Here's the drawing with two shaded views (mm, measured from the low corner). I have some questions. A direction names the side the tool comes from. Round coordinates to 2 decimals unless told otherwise and drop trailing zeros. Order: outer loops, then holes, each group sorted by start corner. A loop starts at its lowest first (then second) coordinate and runs counter-clockwise, first axis right, second up. Notation, with made-up numbers: (49.25, 60.5) -> (78.25, 60.5) arc R14 cw to (78.25, 84.5) -> close; hole circle Ø8 at (-32.75, 36). An arc over 180 degrees is marked (long way). One line per question, with ' | ' between items.
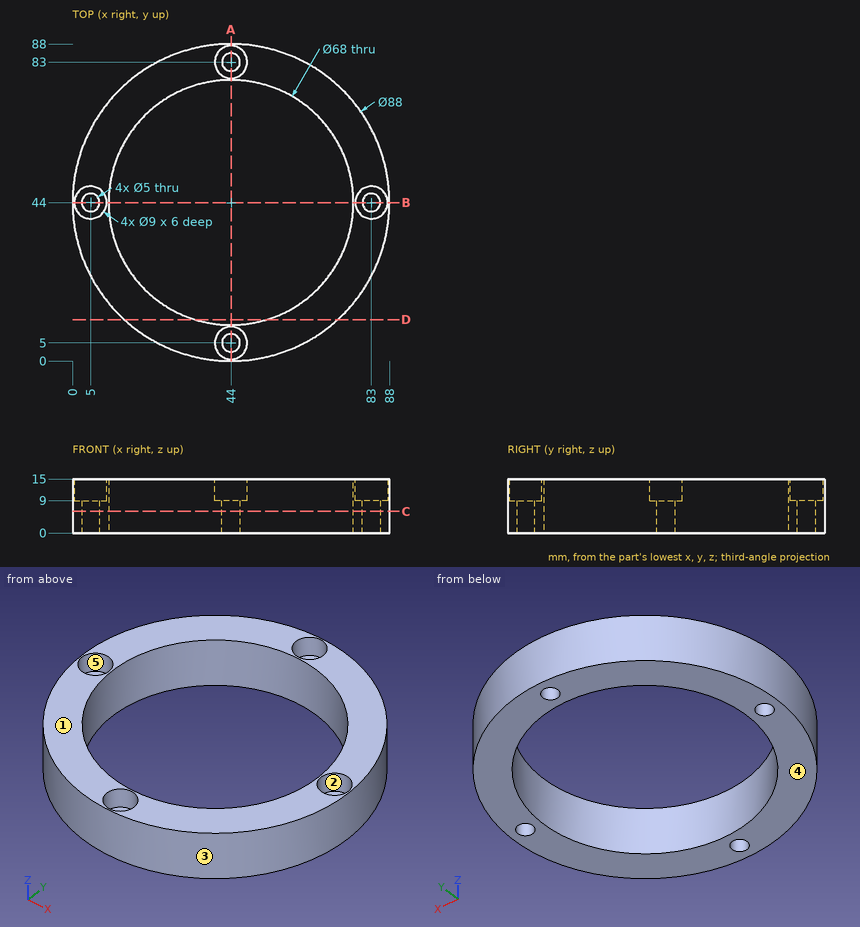
1. If we mould it in two halves opening along X, with no side actions, what happens to the marked faces 3, 4 and 5? For each: pulls with the +X half, pulls with the -X half, needs draft (parallel to the pull), parting line crosses it, or undercut.
From the geometry:
face 3: parting line crosses it | face 4: needs draft | face 5: undercut
2. I'm going to push flat-ended pins straight in: pin 1 (4.5 mm diameter, centred on x = 44.5, y = 85, fed in from +Z); pin 2 (4.5 mm diameter, centred on x = 83, y = 44, fed in from +Z); pin 3 (1 mm diameter, centred on y = 64.5, z = 8, fed in from +X); pin 4 (5 mm diameter, centred on x = 34, z = 6.5, fed in from +Y). Where does each tip first touch, or does it pass through?
From the geometry:
pin 1: stops at z = 9 | pin 2: passes through | pin 3: stops at x = 83.19 | pin 4: stops at y = 87.36
3. I want a section at A-A on x = 44. List the corners of the cut face in (y, z) for me.
From the geometry:
outline: (0, 0) -> (2.5, 0) -> (2.5, 9) -> (0.5, 9) -> (0.5, 15) -> (0, 15) -> close; (7.5, 0) -> (10, 0) -> (10, 15) -> (9.5, 15) -> (9.5, 9) -> (7.5, 9) -> close; (78, 0) -> (80.5, 0) -> (80.5, 9) -> (78.5, 9) -> (78.5, 15) -> (78, 15) -> close; (85.5, 0) -> (88, 0) -> (88, 15) -> (87.5, 15) -> (87.5, 9) -> (85.5, 9) -> close
4. I want a section at C-C on z = 6. List the corners of the cut face in (x, y) for me.
From the geometry:
outline: circle Ø88 at (44, 44); hole circle Ø5 at (5, 44); hole circle Ø68 at (44, 44); hole circle Ø5 at (44, 5); hole circle Ø5 at (44, 83); hole circle Ø5 at (83, 44)
5. On a 3-axis mill with a long thin cutter (end or side, diameter ignored), from which of +Z, -Z, +X, -X, +Y, -Y can I reach the whole of each face in a straight line? I mean the marked faces 1 and 2. Say none if no direction works.
From the geometry:
face 1: +Z, +X, -X, +Y, -Y | face 2: +Z
6. I want a section at D-D on y = 11.5. List the corners of the cut face in (x, z) for me.
From the geometry:
outline: (14.34, 0) -> (34.01, 0) -> (34.01, 15) -> (14.34, 15) -> close; (53.99, 0) -> (73.66, 0) -> (73.66, 15) -> (53.99, 15) -> close
7. I need wall thicknesses on probe 1 along Y at (x, z) = (41.5, 9.75); probe 2 along Y at (x, z) = (43, 0.75); probe 3 along Y at (x, z) = (68, 1). Which ranges of each line are inside material? Lowest first, please.
From the geometry:
probe 1: y = 0.07 to 1.26, 8.74 to 10.09, 77.91 to 79.26, 86.74 to 87.93 | probe 2: y = 0.01 to 2.71, 7.29 to 10.01, 77.99 to 80.71, 85.29 to 87.99 | probe 3: y = 7.12 to 19.92, 68.08 to 80.88
